```python
from build123d import *

# Parameters (mm, degrees)
SKETCH1_R           = 6
SKETCH1_R_2         = 5
BOSS_EXTRUDE1_DEPTH = 20


with BuildPart() as part:
    # Sketch1 → Boss-Extrude1 (new body)
    with BuildSketch(Plane.XY):
        with BuildLine():
            Line((0, 10), (20, 10))
            ThreePointArc((20, 10), (30, 0), (20, -10))
            Line((20, -10), (0, -10))
            Line((0, -10), (0, -30))
            Line((0, -30), (40, -30))
            Line((40, -30), (84.685564793, -11.047419724))
            ThreePointArc((84.685564793, -11.047419724), (92, 0), (84.685564793, 11.047419724))
            Line((84.685564793, 11.047419724), (40, 30))
            Line((40, 30), (0, 30))
            Line((0, 30), (0, 10))
        make_face()
        with Locations((80, 0)):
            Circle(SKETCH1_R, mode=Mode.SUBTRACT)
        with Locations((10, 20)):
            Circle(SKETCH1_R_2, mode=Mode.SUBTRACT)
        with Locations((30, 20)):
            Circle(SKETCH1_R_2, mode=Mode.SUBTRACT)
        with Locations((30, -20)):
            Circle(SKETCH1_R_2, mode=Mode.SUBTRACT)
        with Locations((10, -20)):
            Circle(SKETCH1_R_2, mode=Mode.SUBTRACT)
    extrude(amount=BOSS_EXTRUDE1_DEPTH)


solid = part.part
```
Geometry check sheet. Reference: the model listing, model coordinates, mm. A direction names the side the tool comes from. Coordinates: 2 decimals unless noted, no trailing zeros. Write each loop counter-clockwise with the first axis right and the second up, starting at its lowest first coordinate (ties: lowest second). Pieces come first, ordered by that corner, then holes. Notation, with made-up numbers: (70.25, 9) -> (99.25, 9) arc R6 ccw to (99.25, 18) -> close; hole circle Ø5 at (14.5, 82.5). An arc over 180 degrees is marked (long way). Use CSV: the item, a comma, the result in double quotes. Start each with the question number.
Item 1: Mould release check, pull along X, two halves, no side actions. Record for faces 3 (the flat face through (20, -30, 10)), 4 (the cylindrical face through (26, 17, 10)), 5 (the flat face through (62.66, 20.39, 9.86)): released by +X, released by -X, zero draft, split by the parting line, or undercut.
Item 2: Set-up check for faces 1 (the flat face through (10, 10, 10)), 2 (the cylindrical face through (12.307, -24.436, 9.86)): record each of +Z, -Z, +X, -X, +Y, -Y from which the full face is reachable in a straight line by a thin tool's end or side.
Item 3: Thickness scan on line 1 (Y direction, x = 10, z = 4.75); line 2 (Y direction, x = 9, z = 12.25); line 3 (X direction, y = -17, z = 14). Record the ranges inside material, lowest first.
Item 4: Cross-section at A-A, the plane x = 10. Record the cut outline in (y, z).
Item 5: Cross-section at B-B, the plane y = 0. Record the cut outline in (x, z).
Item 6: Cross-section at C-C, the plane z = 13.5. Record the cut outline in (x, y).
Item 7: Depth check by flat-ended pin: pin 1 Ø10 at (y, z) = (-22, 10.5) entering from +X; pin 2 Ø9.5 at (x, y) = (80, 0) entering from -Z. Enter the tip coordinate at first touch or a pass-through.
Item 8: Cross-section at D-D, the plane x = 80. Record the cut outline in (y, z).
Answers:
1,face 3,"zero draft"
1,face 4,"undercut"
1,face 5,"released by +X"
2,face 1,"+Z, -Z, -X"
2,face 2,"+Z, -Z"
3,line 1,"-30 to -25, -15 to -10, 10 to 15, 25 to 30"
3,line 2,"-30 to -24.9, -15.1 to -10, 10 to 15.1, 24.9 to 30"
3,line 3,"0 to 6, 14 to 26, 34 to 70.65"
4,outline,"(-30, 0) -> (-25, 0) -> (-25, 20) -> (-30, 20) -> close; (-15, 0) -> (-10, 0) -> (-10, 20) -> (-15, 20) -> close; (10, 0) -> (15, 0) -> (15, 20) -> (10, 20) -> close; (25, 0) -> (30, 0) -> (30, 20) -> (25, 20) -> close"
5,outline,"(30, 0) -> (74, 0) -> (74, 20) -> (30, 20) -> close; (86, 0) -> (92, 0) -> (92, 20) -> (86, 20) -> close"
6,outline,"(0, -30) -> (40, -30) -> (84.69, -11.05) arc R12 ccw to (84.69, 11.05) -> (40, 30) -> (0, 30) -> (0, 10) -> (20, 10) arc R10 cw to (20, -10) -> (0, -10) -> close; hole circle Ø10 at (10, -20); hole circle Ø10 at (10, 20); hole circle Ø10 at (30, -20); hole circle Ø10 at (30, 20); hole circle Ø12 at (80, 0)"
7,pin 1,"x = 70.65"
7,pin 2,"through"
8,outline,"(-13.03, 0) -> (-6, 0) -> (-6, 20) -> (-13.03, 20) -> close; (6, 0) -> (13.03, 0) -> (13.03, 20) -> (6, 20) -> close"
